Build history of the part. All positions in model axes, mm. Face numbers are marked on the shaded views. A direction names the side the tool comes from. Coordinates: 2 decimals unless noted, no trailing zeros. Order: outer loops, then holes, each group sorted by start corner. A loop starts at its lowest first (then second) coordinate and runs counter-clockwise, first axis right, second up. Notation, with made-up numbers: (87, 8) - (95, 8) arc R32 ccw to (95, 34) - close; hole circle Ø6 at (24, -10). An arc over 180 degrees is marked (long way). Return JSON: item names as keys, results as strings.
from build123d import *

# Parameters (mm, degrees)
F0_W          = 15
F0_H          = 8.75
F0_H_2        = 17.5
F1_DEPTH      = 40
F2_DEPTH      = 55
F3_DEPTH      = 15
F7_DEPTH      = 20.4590409994
F8_ANGLE      = 180
F10_DEPTH     = 25
F11_T4_DEPTH  = 56.0752448195
F11_T12_DEPTH = 56.0752448195
F11_T20_DEPTH = 56.0752448195
F11_T28_DEPTH = 56.0752448195


# Not quite as in the source:
# - a fillet or chamfer that OpenCascade refuses, or shapes differently, is made with other operations: its cross-section is extruded or revolved along the edge and cut away or added


with BuildPart() as f1:
    # F0 (on Top) → F1 (new body)
    with BuildSketch(Plane.XY):
        with Locations((0, 13.125)):
            Rectangle(F0_W, F0_H)
        with Locations((0, -8.75)):
            Rectangle(F0_W, F0_H_2)
        with Locations((0, 4.375)):
            Rectangle(F0_W, F0_H)
        with Locations((15, 13.125)):
            Rectangle(F0_W, F0_H)
        Polygon((22.5, 8.75), (7.5, 8.75), (7.5, 0), align=None)
        with Locations((-15, 13.125)):
            Rectangle(F0_W, F0_H)
        Polygon((-7.5, 0), (-7.5, 8.75), (-22.5, 8.75), align=None)
    extrude(amount=F1_DEPTH)



with BuildPart() as f2:
    # F0 (on Top) → F2 (new body)
    with BuildSketch(Plane.XY):
        with Locations((0, 4.375)):
            Rectangle(F0_W, F0_H)
        with Locations((0, 13.125)):
            Rectangle(F0_W, F0_H)
    extrude(amount=F2_DEPTH)


with BuildPart() as f1_1:
    add(f1.part)

    add(f2.part)  # F3 merges F2
    # F0 (on Top) → F3 (join)
    with BuildSketch(Plane.XY):
        with Locations((0, 4.375)):
            Rectangle(F0_W, F0_H)
        with Locations((0, 13.125)):
            Rectangle(F0_W, F0_H)
    extrude(amount=-F3_DEPTH)

    # F4: union 


with BuildPart() as f1_2:
    # F6: moved
    add(f1_1.part.moved(Location((7.5, 0, 0))))

    # F5 (on Right) → F7 (cut)
    with BuildSketch(Plane.YZ):
        Polygon((8.75, -15), (0, 0), (0, -15), align=None)
    extrude(amount=F7_DEPTH, mode=Mode.SUBTRACT)


with BuildPart() as f1_3:
    # F8: moved
    add(f1_2.part.rotate(Axis((7.5, 0, 0), (0, -1, 0)), F8_ANGLE))


with BuildPart() as f1_4:
    # F9: moved
    add(f1_3.part.moved(Location((0, 0, 40))))

    # F5 (on Right) → F10 (cut)
    with BuildSketch(Plane.YZ):
        Polygon((8.75, -15), (0, 0), (0, -15), align=None)
    extrude(amount=F10_DEPTH, mode=Mode.SUBTRACT)

    # F11: chamfer of 15 on 4 edges, made by hand


with BuildPart() as f11_tool2:
    # F11_s3 → F11_t4 (new body)
    with BuildSketch(Plane.XZ.offset(-17.5)):
        Polygon((30, 40), (15, 55), (15, 40), align=None)
    extrude(amount=F11_T4_DEPTH)

    split(bisect_by=Plane.YZ.offset(30), keep=Keep.BOTTOM)

    split(bisect_by=Plane(origin=(3.8082901554, -6.5284974093, 0), x_dir=(0, 0, 1), z_dir=(-0.5038710255, 0.8637789009, 0)), keep=Keep.TOP)

    split(bisect_by=Plane(origin=(0, -17.4093264249, 10.1554404145), x_dir=(1, 0, 0), z_dir=(0, 0.8637789009, -0.5038710255)), keep=Keep.TOP)

    split(bisect_by=Plane.XY.offset(55), keep=Keep.BOTTOM)


with BuildPart() as f1_5:
    add(f1_4.part)

    # F11_t1: union F11_tool2
    add(f11_tool2.part)


with BuildPart() as f11_tool10:
    # F11_s11 → F11_t12 (new body)
    with BuildSketch(Plane.XZ.offset(38.5752448195)):
        Polygon((-15, 0), (0, -15), (0, 0), align=None)
    extrude(amount=-F11_T12_DEPTH)

    split(bisect_by=Plane.YZ.offset(-15), keep=Keep.TOP)

    split(bisect_by=Plane(origin=(0, 0, 0), x_dir=(0, 0, 1), z_dir=(0.5038710255, 0.8637789009, 0)), keep=Keep.TOP)

    split(bisect_by=Plane.XY.offset(-15), keep=Keep.TOP)

    split(bisect_by=Plane(origin=(0, 0, 0), x_dir=(1, 0, 0), z_dir=(0, 0.8637789009, 0.5038710255)), keep=Keep.TOP)


with BuildPart() as f1_6:
    add(f1_5.part)

    # F11_t9: union F11_tool10
    add(f11_tool10.part)


with BuildPart() as f11_tool18:
    # F11_s19 → F11_t20 (new body)
    with BuildSketch(Plane.XZ.offset(-17.5)):
        Polygon((15, -15), (30, 0), (15, 0), align=None)
    extrude(amount=F11_T20_DEPTH)

    split(bisect_by=Plane.XY.offset(-15), keep=Keep.TOP)

    split(bisect_by=Plane(origin=(0, 0, 0), x_dir=(1, 0, 0), z_dir=(0, 0.8637789009, 0.5038710255)), keep=Keep.TOP)

    split(bisect_by=Plane(origin=(3.8082901554, -6.5284974093, 0), x_dir=(0, 0, 1), z_dir=(-0.5038710255, 0.8637789009, 0)), keep=Keep.TOP)

    split(bisect_by=Plane.YZ.offset(30), keep=Keep.BOTTOM)


with BuildPart() as f1_7:
    add(f1_6.part)

    # F11_t17: union F11_tool18
    add(f11_tool18.part)


with BuildPart() as f11_tool26:
    # F11_s27 → F11_t28 (new body)
    with BuildSketch(Plane.XZ.offset(38.5752448195)):
        Polygon((0, 55), (-15, 40), (0, 40), align=None)
    extrude(amount=-F11_T28_DEPTH)

    split(bisect_by=Plane.XY.offset(55), keep=Keep.BOTTOM)

    split(bisect_by=Plane(origin=(0, -17.4093264249, 10.1554404145), x_dir=(1, 0, 0), z_dir=(0, 0.8637789009, -0.5038710255)), keep=Keep.TOP)

    split(bisect_by=Plane.YZ.offset(-15), keep=Keep.TOP)

    split(bisect_by=Plane(origin=(0, 0, 0), x_dir=(0, 0, 1), z_dir=(0.5038710255, 0.8637789009, 0)), keep=Keep.TOP)


with BuildPart() as f1_8:
    add(f1_7.part)

    # F11_t25: union F11_tool26
    add(f11_tool26.part)


solid = f1_8.part
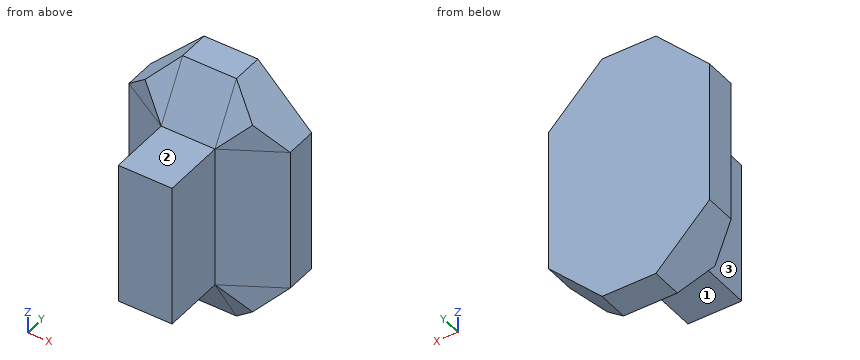
1. Cut at C-C on y = -6. Give the cut face in (x, z), plus the area to 3 significant figures.
Check values:
{"outline": "(0, 0) - (15, 0) - (15, 40) - (0, 40) - close", "area": "600 mm²"}
2. Tool access for the marked faces 1, 2 and 3: list every direction of +Z, -Z, +X, -X, +Y, -Y with a clear straight run to the whole face (end or side of a thin tool).
Check values:
{"face 1": "-Z, +X, -X, -Y", "face 2": "+Z, +X, -X, -Y", "face 3": "+Z, -Z, -X, -Y"}
3. Cut at A-A on x = -3. Give the cut face in (y, z).
Check values:
{"outline": "(1.75, -3) - (7, -12) - (17.5, -12) - (17.5, 52) - (7, 52) - (1.75, 43) - close"}
4. Probe L1, parallel to Z at x = 13, y = -7; L2, parallel to Y at x = 22.5, z = 36 (3 decimals); L3, parallel to X at y = -4, z = 20.5. List the from-to ranges inside material, lowest first.
Check values:
{"L1": "0 to 40", "L2": "4.375 to 17.5", "L3": "0 to 15"}
5. Drop flat-ended pins along their axis: pin 1 (2 mm diameter, centred on x = 5.5, y = -14, fed in from -Z); pin 2 (6 mm diameter, centred on y = 0.5, z = -3.5, fed in from -X); pin 3 (4.5 mm diameter, centred on x = 10.5, y = -10.5, fed in from +Z); pin 4 (3 mm diameter, centred on x = 15.5, z = 18.5, fed in from -Y). Give the stop position or say it passes through.
Check values:
{"pin 1": "z = 0", "pin 2": "x = -6", "pin 3": "z = 40", "pin 4": "y = -17.5"}
6. Cut at B-B on z = 1.5. Give the cut face in (x, y), plus the area to 3 significant figures.
Check values:
{"outline": "(-15, 8.75) - (0, 0) - (0, -17.5) - (15, -17.5) - (15, 0) - (30, 8.75) - (30, 17.5) - (-15, 17.5) - close", "area": "919 mm²"}
7. Cut at D-D on z = 50. Give the cut face in (x, y), plus the area to 3 significant figures.
Check values:
{"outline": "(-5, 5.83) - (20, 5.83) - (20, 17.5) - (-5, 17.5) - close", "area": "292 mm²"}
